from build123d import *

# Parameters (mm, degrees)
ESQUISSE1_W             = 50
ESQUISSE1_H             = 41
ESQUISSE1_R             = 1.65
ESQUISSE1_R_2           = 3
BOSS_EXTRU_1_DEPTH      = 26
ESQUISSE2_W             = 20
ESQUISSE2_H             = 17
ENL_V_MAT_EXTRU_1_DEPTH = 51
ESQUISSE3_R             = 9
ENL_V_MAT_EXTRU_2_DEPTH = 19.5
ESQUISSE3_3_R           = 1.3
ENL_V_MAT_EXTRU_3_DEPTH = 15
ESQUISSE1_3_R           = 1.65
ENL_V_MAT_EXTRU_4_DEPTH = 11
ESQUISSE4_R             = 7
ENL_V_MAT_EXTRU_5_DEPTH = 51.0000001
ESQUISSE4_3_R           = 9
ENL_V_MAT_EXTRU_6_DEPTH = 13
ESQUISSE4_4_R           = 7.5
ENL_V_MAT_EXTRU_7_DEPTH = 23


with BuildPart() as part:
    # Esquisse1 → Boss.-Extru.1 (new body)
    with BuildSketch(Plane(origin=(0, 0, 0), x_dir=(1, 0, 0), z_dir=(0, 1, 0))):
        with Locations((-25, 20.5)):
            Rectangle(ESQUISSE1_W, ESQUISSE1_H)
        with Locations((-45, 18.35)):
            Circle(ESQUISSE1_R, mode=Mode.SUBTRACT)
        with Locations((-5, 18.35)):
            Circle(ESQUISSE1_R, mode=Mode.SUBTRACT)
        with Locations(Location((-5, 32.5, 0), (0, 0, 270))):  # turned: the seam where the file's is
            Circle(ESQUISSE1_R_2, mode=Mode.SUBTRACT)
        with Locations(Location((-45, 32.5, 0), (0, 0, 270))):  # turned: the seam where the file's is
            Circle(ESQUISSE1_R_2, mode=Mode.SUBTRACT)
        with Locations((-45, 18.35)):
            Circle(ESQUISSE1_R)
        with Locations((-5, 18.35)):
            Circle(ESQUISSE1_R)
    extrude(amount=BOSS_EXTRU_1_DEPTH)

    # Esquisse2 → Enl_v. mat.-Extru.1 (cut, through all)
    with BuildSketch(Plane(origin=(0, 0, 0), x_dir=(0, 0, -1), z_dir=(1, 0, 0))):
        with Locations((31, 17.5)):
            Rectangle(ESQUISSE2_W, ESQUISSE2_H)
    extrude(amount=-ENL_V_MAT_EXTRU_1_DEPTH, mode=Mode.SUBTRACT)

    # Esquisse3 → Enl_v. mat.-Extru.2 (cut)
    with BuildSketch(Plane(origin=(0, 0, 0), x_dir=(0, 0, -1), z_dir=(1, 0, 0))):
        with Locations((10.5, 14.8)):
            Circle(ESQUISSE3_R)
    extrude(amount=-ENL_V_MAT_EXTRU_2_DEPTH, mode=Mode.SUBTRACT)

    # Esquisse3_3 → Enl_v. mat.-Extru.3 (cut)
    with BuildSketch(Plane(origin=(0, 0, 0), x_dir=(0, 0, -1), z_dir=(1, 0, 0))):
        with Locations((2.5, 6.5)):
            Circle(ESQUISSE3_3_R)
        with Locations((18.5, 6.5)):
            Circle(ESQUISSE3_3_R)
    extrude(amount=-ENL_V_MAT_EXTRU_3_DEPTH, mode=Mode.SUBTRACT)

    # Esquisse1_3 → Enl_v. mat.-Extru.4 (cut)
    with BuildSketch(Plane(origin=(0, 0, 0), x_dir=(1, 0, 0), z_dir=(0, 1, 0))):
        with Locations(Location((-5, 18.35, 0), (0, 0, 169.22643943))):  # turned: the seam where the file's is
            Circle(ESQUISSE1_3_R)
        with Locations(Location((-45, 18.35, 0), (0, 0, 270))):  # turned: the seam where the file's is
            Circle(ESQUISSE1_3_R)
    extrude(amount=ENL_V_MAT_EXTRU_4_DEPTH, mode=Mode.SUBTRACT)

    # Esquisse4 → Enl_v. mat.-Extru.5 (cut, through all)
    with BuildSketch(Plane.ZY.offset(50)):
        with Locations((-10.5, 14.8)):
            Circle(ESQUISSE4_R)
    extrude(amount=-ENL_V_MAT_EXTRU_5_DEPTH, mode=Mode.SUBTRACT)

    # Esquisse4_3 → Enl_v. mat.-Extru.6 (cut)
    with BuildSketch(Plane.ZY.offset(50)):
        with Locations(Location((-10.5, 14.8, 0), (0, 0, 180))):  # turned: the seam where the file's is
            Circle(ESQUISSE4_3_R)
    extrude(amount=-ENL_V_MAT_EXTRU_6_DEPTH, mode=Mode.SUBTRACT)

    # Esquisse4_4 → Enl_v. mat.-Extru.7 (cut)
    with BuildSketch(Plane.ZY.offset(50)):
        with Locations((-10.5, 14.8)):
            Circle(ESQUISSE4_4_R)
    extrude(amount=-ENL_V_MAT_EXTRU_7_DEPTH, mode=Mode.SUBTRACT)


solid = part.part
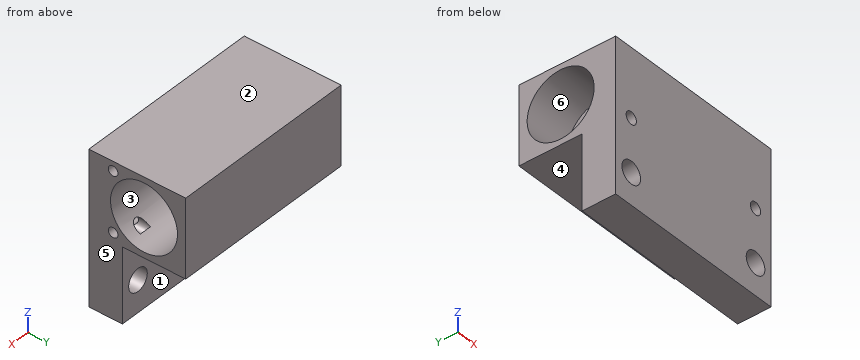
Model file for the job. Use its own axes, mm. Face numbers are marked on the shaded views. A direction names the side the tool comes from. Round coordinates to 2 decimals unless told otherwise and drop trailing zeros. Order: outer loops, then holes, each group sorted by start corner. A loop starts at its lowest first (then second) coordinate and runs counter-clockwise, first axis right, second up. Notation, with made-up numbers: M 8.25,89 L 14.25,89 A15 cw 14.25,113 Z; hole C 73,71 d8. An arc over 180 degrees is marked long. Write each question's results on one line, items separated by ' | '. Start each with the question number.
(1) Saw through at A-A, the plane z = -10.5. Give the cut face in (x, y), then the cut area to 3 significant figures.
(2) Saw through at D-D, the plane z = -32. Give the cut face in (x, y).
(3) Which spindle directions (+Z, -Z, +X, -X, +Y, -Y) get a long thin tool onto all of the face, cutting with end or side? Do the marked faces 1, 2 and 3. Say none if no direction does.
(4) Drop flat-ended pins along their axis: pin 1 (1.1 mm diameter, centred on x = -4.5, z = -19, fed in from -Y); pin 2 (4.5 mm diameter, centred on y = 11.5, z = -9.5, fed in from -X); pin 3 (14.5 mm diameter, centred on y = 14.8, z = -10.5, fed in from +X); pin 4 (8.5 mm diameter, centred on x = -24.5, y = 14.5, fed in from -Z). Give the stop position or say it passes through.
(5) Probe probe 1 along X at (y, z) = (2, -32.5); probe 2 along Z at (x, y) = (-5, 4.75); probe 3 along X at (y, z) = (3.75, -18). List the from-to ranges inside material, lowest first. Write a range as from..to.
(6) Saw through at B-B, the plane y = 14.8. Give the cut face in (x, z), then the cut area to 3 significant figures.
(7) Saw through at C-C, the plane x = -16. Give the cut face in (y, z), then the cut area to 3 significant figures.
(8) Two-plate mould, pull along Z, no slides. Class the marked faces 4, 5 and 6: pulls with the +Z half, pulls with the -Z half, needs draft (parallel to the pull), parting line crosses it, or undercut.
Established:
1) outline: M -50,0 L 0,0 L 0,5.8 L -19.5,5.8 L -19.5,7.8 L -27,7.8 L -27,7.3 L -37,7.3 L -37,5.8 L -50,5.8 Z; M -50,23.8 L -37,23.8 L -37,22.3 L -27,22.3 L -27,21.8 L -19.5,21.8 L -19.5,23.8 L 0,23.8 L 0,26 L -50,26 Z | area: 460 mm^2
2) outline: M -50,0 L -47.96,0 L -47.96,9 L -50,9 Z; M -42.04,0 L -7.96,0 L -7.96,9 L -42.04,9 Z; M -2.04,0 L 0,0 L 0,9 L -2.04,9 Z
3) face 1: -Z, +X, -X, +Y | face 2: +Z, +X, -X, +Y, -Y | face 3: +X
4) pin 1: stops at y = 11 | pin 2: passes through | pin 3: stops at x = -19.5 | pin 4: stops at z = -21
5) probe 1: x = -50..-48, -42..-8, -2..0 | probe 2: z = -41..-35.5, -29.5..-20, -16.7..0 | probe 3: x = -50..-46.61, -43.39..-6.61, -3.39..0
6) outline: M -50,-21 L 0,-21 L 0,-19.5 L -19.5,-19.5 L -19.5,-17.5 L -27,-17.5 L -27,-18 L -37,-18 L -37,-19.5 L -50,-19.5 Z; M -50,-1.5 L -37,-1.5 L -37,-3 L -27,-3 L -27,-3.5 L -19.5,-3.5 L -19.5,-1.5 L 0,-1.5 L 0,0 L -50,0 Z | area: 210 mm^2
7) outline: M 0,-41 L 9,-41 L 9,-21 L 26,-21 L 26,0 L 0,0 Z; hole C 14.8,-10.5 d18 | area: 472 mm^2
8) face 4: pulls with the -Z half | face 5: needs draft | face 6: undercut
